Could you check a few things on this drawing? It's one solid part, dimensions in mm from its lowest x, y, z. Give positions to 0.01 mm unless a question says otherwise; leave off trailing zeros. Write each loop counter-clockwise with the first axis right and the second up, starting at its lowest first coordinate (ties: lowest second). Pieces come first, ordered by that corner, then holes. Notation, with made-up numbers: M 35.5,-32 L 44.5,-32 A13 ccw 44.5,-7 Z; hole C -12.75,10.25 d9. An arc over 180 degrees is marked long. Write each question's results on one line, items separated by ' | '.
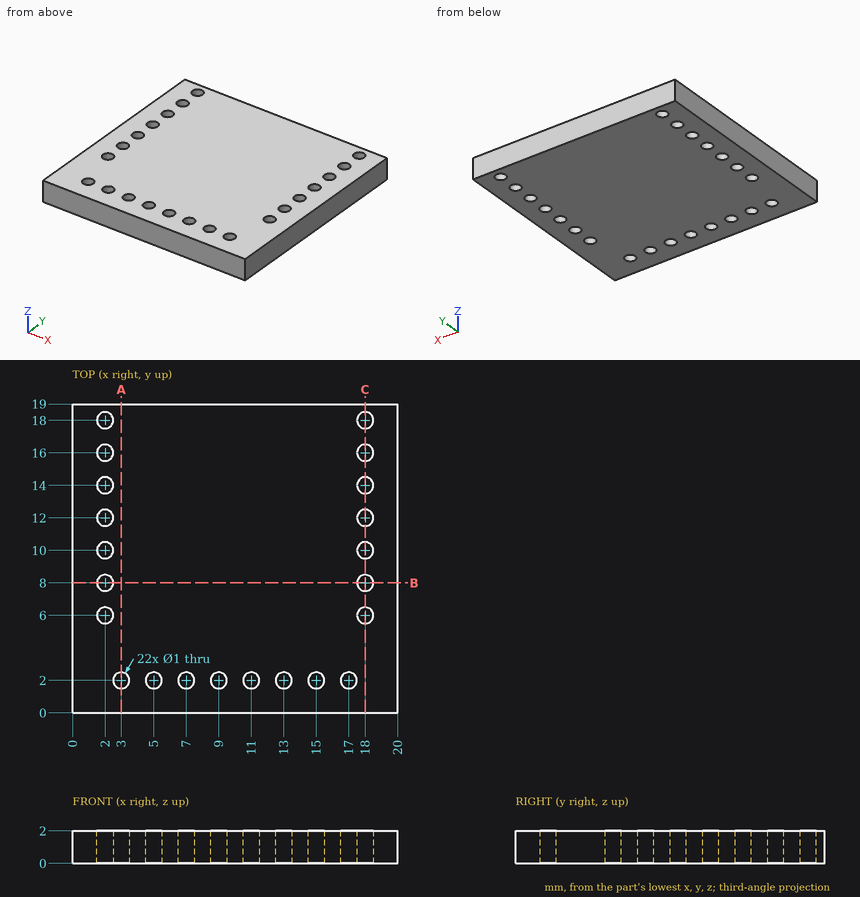
Item 1: I want a section at A-A, the plane x = 3. Please give me the cut outline in (y, z).
Geometry says:
outline: M 0,0 L 1.5,0 L 1.5,2 L 0,2 Z; M 2.5,0 L 19,0 L 19,2 L 2.5,2 Z
Item 2: I want a section at C-C, the plane x = 18. Give the number of separate pieces and of enclosed holes in the cut face, and give its area (3 significant figures).
Geometry says:
separate pieces: 8 | enclosed holes: 0 | area: 24.0 mm2
Item 3: If I drill on line 1 (X direction, y = 18, z = 0.65); line 2 (Y direction, x = 17, z = 0.7); line 3 (X direction, y = 10.25, z = 1.65), over which ranges is the centre line in solid material (lowest first)? Write a range as from..to.
Geometry says:
line 1: x = 0..1.5, 2.5..17.5, 18.5..20 | line 2: y = 0..1.5, 2.5..19 | line 3: x = 0..1.57, 2.43..17.57, 18.43..20
Item 4: I want a section at B-B, the plane y = 8. Please give me the cut outline in (x, z).
Geometry says:
outline: M 0,0 L 1.5,0 L 1.5,2 L 0,2 Z; M 2.5,0 L 17.5,0 L 17.5,2 L 2.5,2 Z; M 18.5,0 L 20,0 L 20,2 L 18.5,2 Z
